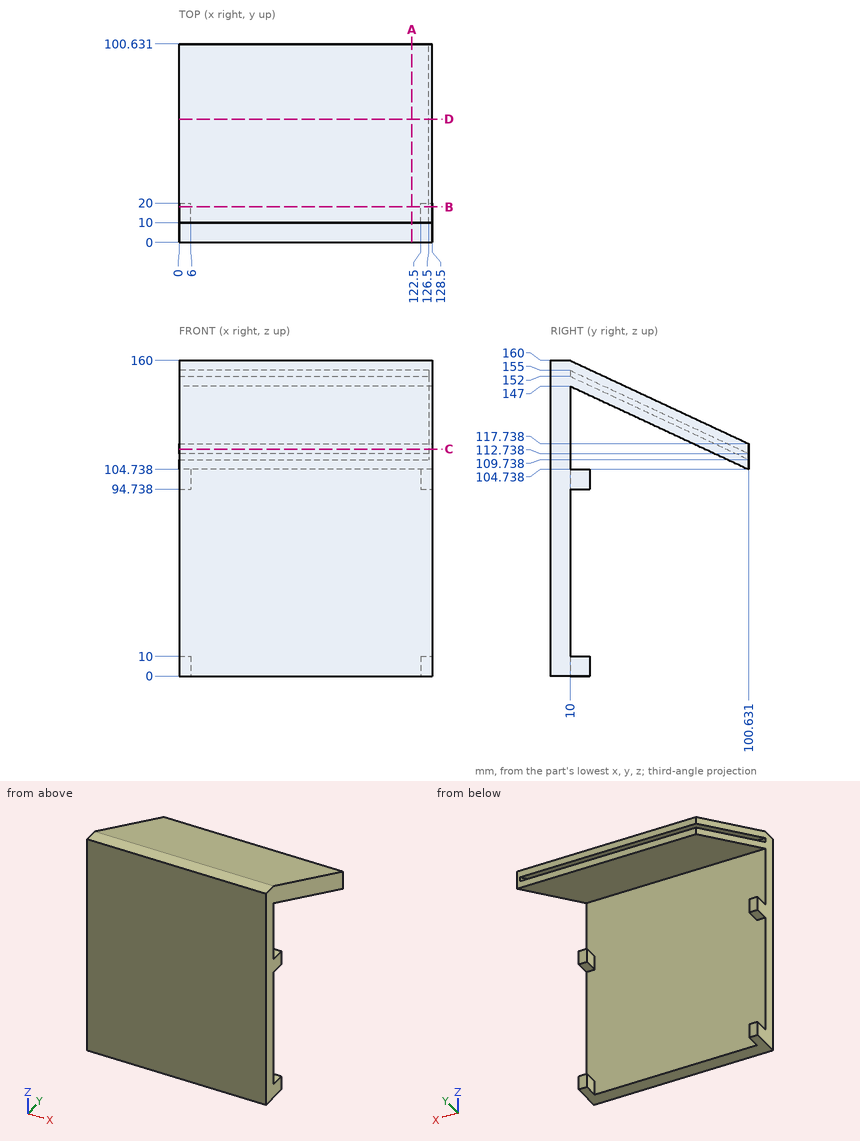
Could you check a few things on this drawing? It's one solid part, dimensions in mm from its lowest x, y, z. Round coordinates to 2 decimals unless told otherwise and drop trailing zeros. Order: outer loops, then holes, each group sorted by start corner. A loop starts at its lowest first (then second) coordinate and runs counter-clockwise, first axis right, second up. Notation, with made-up numbers: M 6,-4 L 41,-4 A15 ccw 41,23 Z; hole C -35.75,18.5 d2. An arc over 180 degrees is marked long. One line per item, written item: value.
(1) Imagine slicing it at D-D (y = 62.5). Write out the boundary of the cut face in (x, z).
Ans:
outline: M 0,122.52 L 128.5,122.52 L 128.5,135.52 L 0,135.52 L 0,130.52 L 126.5,130.52 L 126.5,127.52 L 0,127.52 Z
(2) Imagine slicing it at C-C (z = 115). Write out the boundary of the cut face in (x, y), and give its area (3 significant figures).
Ans:
outline: M 0,0 L 128.5,0 L 128.5,10 L 0,10 Z; M 0,78.62 L 128.5,78.62 L 128.5,100.63 L 0,100.63 L 0,95.78 L 126.5,95.78 L 126.5,89.35 L 0,89.35 Z
area: 3,300 mm^2
(3) I need wall thicknesses on line 1 along Y through (x, z) = (40.5, 139.5) (1 decimal); line 2 along Y through (x, z) = (95, 136) (1 decimal); line 3 along Y through (x, z) = (34, 40). Which ranges of each line are inside material? Lowest first, please. Write a range as from..to.
Ans:
line 1: y = 0..10, 26.1..36.8, 43.2..54
line 2: y = 0..10, 33.6..44.3, 50.7..61.5
line 3: y = 0..10
(4) I'm going to push flat-ended pins straight in: P1, Ø8, axis at x = 93, z = 111, coming from the +Y side; P2, Ø5, axis at x = 126, y = 15, coming from the +Z side; P3, Ø2, axis at x = 80, y = 33.5, coming from the +Z side; P4, Ø5, axis at x = 124, y = 16, coming from the +Z side. Where does each tip first touch, or does it pass through?
Ans:
P1: stops at y = 100.63
P2: stops at z = 158.83
P3: stops at z = 149.51
P4: stops at z = 158.37
(5) Imagine slicing it at B-B (y = 18). Write out the boundary of the cut face in (x, z).
Ans:
outline: M 0,0 L 6,0 L 6,10 L 0,10 Z; M 0,94.74 L 6,94.74 L 6,104.74 L 0,104.74 Z; M 0,143.27 L 128.5,143.27 L 128.5,156.27 L 0,156.27 L 0,151.27 L 126.5,151.27 L 126.5,148.27 L 0,148.27 Z; M 122.5,0 L 128.5,0 L 128.5,10 L 122.5,10 Z; M 122.5,94.74 L 128.5,94.74 L 128.5,104.74 L 122.5,104.74 Z
(6) Imagine slicing it at A-A (x = 118). Write out the boundary of the cut face in (y, z), and give its area (3 significant figures).
Ans:
outline: M 0,0 L 10,0 L 10,147 L 100.63,104.74 L 100.63,109.74 L 10,152 L 10,155 L 100.63,112.74 L 100.63,117.74 L 10,160 L 0,160 Z
area: 2,510 mm^2
